Geometry: final body of the model. Coordinates: model frame, mm. A direction names the side the tool comes from. Coordinates: 2 decimals unless noted, no trailing zeros. Write each loop counter-clockwise with the first axis right and the second up, starting at its lowest first coordinate (ties: lowest second). Pieces come first, ordered by that corner, then holes. Notation, with made-up numbers: (33, -34) - (62, -34) arc R24 ccw to (62, 3) - close; hole circle Ø1 at (67, 43.5). An arc over 180 degrees is marked (long way). Answer as a JSON object with one key per item and string values. Group by question number.
Item 1: Mould query, pull axis Y, two halves, no side actions, for faces 3 (the cylindrical face through (-3.675, 22.322, -24.042)), 4 (the flat face through (-149, 21, -27)), 5 (the cylindrical face through (-334.67, -6.174, -24.042)). Classes: pulls with the +Y half, pulls with the -Y half, needs draft (parallel to the pull), parting line crosses it, or undercut.
Item 2: Set-up query: faces 1 (the flat face through (-159, 19.5, -24)), 2 (the flat face through (-149, 21, -21)). Return all of +Z, -Z, +X, -X, +Y, -Y with unobstructed straight access to the full face (end or side cutting, diameter ignored); none if empty.
Item 3: Line query: line 1 along Y through (x, z) = (-209, -21.25); line 2 along Y through (x, z) = (-311.5, -25.1); line 3 along X through (y, z) = (48, -23.4). Output: solid intervals per line, ascending. Write a range as from..to.
Item 4: First-contact query: pin 1 Ø1.5 at (y, z) = (47.5, -23) entering from -X; pin 2 Ø2 at (y, z) = (63.5, -25) entering from -X; pin 3 Ø1.5 at (y, z) = (51.5, -22.5) entering from -X. Flat tips, straight axial feed; report the tip coordinate or a pass-through.
Item 5: Section D-D on y = 40. Return loops of the section in (x, z), and give its area (3 significant figures).
Item 6: Section C-C on y = -2. Return loops of the section in (x, z).
Item 7: Section B-B on z = -22.8. Return loops of the section in (x, y), and give its area (3 significant figures).
Item 8: Section A-A on x = -58. Return loops of the section in (y, z), and give its area (3 significant figures).
Solid Edge part; units mm, degrees
sketch "Sketch1" plane through (0, 0, -27) normal (0, 0, 1) x (1, 0, 0)
  line L0 (-304, 19.5) -> (-10, 19.5)
  line L1 (-1.5304, 28.7183) -> (-5.0835, 70.6112)
  line L2 (4.0714, 71.512) -> (11.9192, 1.447)
  line L3 (-1, -13) -> (-321, -13)
  line L4 (-320.8089, 19.1759) -> (-330.4687, 8.9075)
  line L5 (-318.502, 24.8166) -> (-317.9985, 48.1403)
  line L6 (-305.5643, 45.3509) -> (-311.762, 31.4642)
  arc A0 (-1.5304, 28.7183) -> (-10, 19.5) centre (-10, 28) cw
  arc A1 (4.0714, 71.512) -> (-5.0835, 70.6112) centre (-0.5, 71) ccw
  arc A2 (-1, -13) -> (11.9192, 1.447) centre (-1, 0) ccw
  arc A3 (-321, -13) -> (-330.4687, 8.9075) centre (-321, 0) cw
  arc A4 (-318.502, 24.8166) -> (-320.8089, 19.1759) centre (-327, 25) cw
  arc A5 (-305.5643, 45.3509) -> (-317.9985, 48.1403) centre (-311.5, 48) ccw
  arc A6 (-304, 19.5) -> (-311.762, 31.4642) centre (-304, 28) cw
  line L7 (-10, 21.5) -> (-304, 21.5)
  arc A7 (-304, 21.5) -> (-309.9357, 30.6491) centre (-304, 28) cw
  line L8 (-309.9357, 30.6491) -> (-303.738, 44.5358)
  arc A8 (-303.738, 44.5358) -> (-319.998, 48.1834) centre (-311.5, 48) ccw
  line L9 (-319.998, 48.1834) -> (-320.5015, 24.8597)
  arc A9 (-320.5015, 24.8597) -> (-322.2657, 20.5462) centre (-327, 25) cw
  line L10 (-322.2657, 20.5462) -> (-331.9254, 10.2779)
  arc A10 (-331.9254, 10.2779) -> (-321, -15) centre (-321, 0) ccw
  line L11 (-321, -15) -> (-1, -15)
  arc A11 (-1, -15) -> (13.9068, 1.6697) centre (-1, 0) ccw
  line L12 (13.9068, 1.6697) -> (6.059, 71.7347)
  arc A12 (6.059, 71.7347) -> (-7.0764, 70.4422) centre (-0.5, 71) ccw
  line L13 (-7.0764, 70.4422) -> (-3.5233, 28.5493)
  arc A13 (-3.5233, 28.5493) -> (-10, 21.5) centre (-10, 28) cw
extrude "Protrusion1" add sketch "Sketch1" along normal blind 6
properties material "PVC"
Checks:
{
 "1": {"face 3": "undercut", "face 4": "needs draft", "face 5": "parting line crosses it"},
 "2": {"face 1": "+Z, -Z", "face 2": "+Z, +X, -X, +Y, -Y"},
 "3": {"line 1": "-15..-13, 19.5..21.5", "line 2": "-15..-13, 24..32.05, 54.5..56.5", "line 3": "-320..-318, -305..-303, -5.17..-3.17, 6.7..8.72"},
 "4": {"pin 1": "x = -320.03", "pin 2": "x = -6.57", "pin 3": "x = -319.54"},
 "5": {"outline": "(-320.17, -27) - (-318.17, -27) - (-318.17, -21) - (-320.17, -21) - close; (-307.95, -27) - (-305.76, -27) - (-305.76, -21) - (-307.95, -21) - close; (-4.49, -27) - (-2.49, -27) - (-2.49, -21) - (-4.49, -21) - close; (7.6, -27) - (9.61, -27) - (9.61, -21) - (7.6, -21) - close", "area": "49.3 mm^2"},
 "6": {"outline": "(-335.87, -27) - (-333.85, -27) - (-333.85, -21) - (-335.87, -21) - close; (11.85, -27) - (13.87, -27) - (13.87, -21) - (11.85, -21) - close"},
 "7": {"outline": "(-331.93, 10.28) arc R15 ccw to (-321, -15) - (-1, -15) arc R15 ccw to (13.91, 1.67) - (6.06, 71.73) arc R6.6 ccw to (-7.08, 70.44) - (-3.52, 28.55) arc R6.5 cw to (-10, 21.5) - (-304, 21.5) arc R6.5 cw to (-309.94, 30.65) - (-303.74, 44.54) arc R8.5 ccw (long way) to (-320, 48.18) - (-320.5, 24.86) arc R6.5 cw to (-322.27, 20.55) - close; hole (-330.47, 8.91) arc R13 ccw to (-321, -13) - (-1, -13) arc R13 ccw to (11.92, 1.45) - (4.07, 71.51) arc R4.6 ccw to (-5.08, 70.61) - (-1.53, 28.72) arc R8.5 cw to (-10, 19.5) - (-304, 19.5) arc R8.5 cw to (-311.76, 31.46) - (-305.56, 45.35) arc R6.5 ccw (long way) to (-318, 48.14) - (-318.5, 24.82) arc R8.5 cw to (-320.81, 19.18) - close", "area": "1,820 mm^2"},
 "8": {"outline": "(-15, -27) - (-13, -27) - (-13, -21) - (-15, -21) - close; (19.5, -27) - (21.5, -27) - (21.5, -21) - (19.5, -21) - close", "area": "24.0 mm^2"}
}
